from build123d import *

# Parameters (mm, degrees)
F0_W     = 50.8
F0_H     = 25.4
F2_DEPTH = 25.4
F3_DEPTH = 6.35


with BuildPart() as f2:
    # F0 (on Front) → F2 (new body, symmetric)
    with BuildSketch(Plane.XZ):
        Rectangle(F0_W, F0_H)
    extrude(amount=F2_DEPTH, both=True)

    # F1 (on Front) → F3 (cut, symmetric)
    with BuildSketch(Plane.XZ):
        with BuildLine():
            Line((18.556945, 13.312588), (-18.556941, 13.312588))
            ThreePointArc((-18.556941, 13.312588), (2e-06, 0.164781), (18.556945, 13.312588))
        make_face()
    extrude(amount=F3_DEPTH, both=True, mode=Mode.SUBTRACT)


solid = f2.part
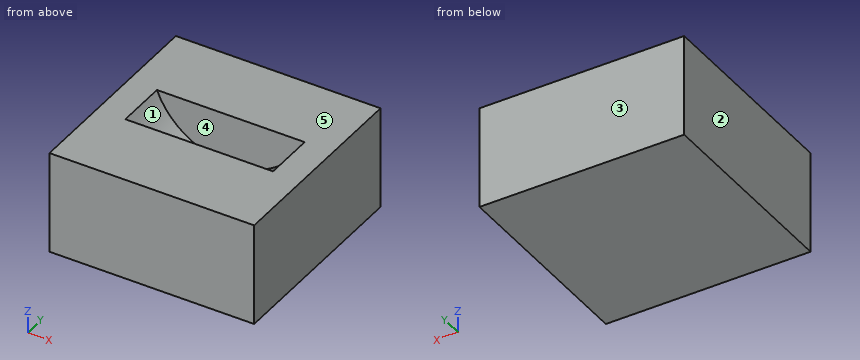
Geometry: final body of the model. Coordinates: model frame, mm. Face numbers are marked on the shaded views. A direction names the side the tool comes from. Round coordinates to 2 decimals unless told otherwise and drop trailing zeros. Order: outer loops, then holes, each group sorted by start corner. A loop starts at its lowest first (then second) coordinate and runs counter-clockwise, first axis right, second up.
Q1. Section C-C, the plane y = 1. Output: boundary loops of the cut face in (x, z).
Result sheet:
outline: (-25.4, -12.7) - (25.4, -12.7) - (25.4, 12.7) - (18.33, 12.7) arc R19.67 cw to (-18.33, 12.7) - (-25.4, 12.7) - close
Q2. Section A-A, the plane z = 11.25. Output: boundary loops of the cut face in (x, y).
Result sheet:
outline: (-25.4, -25.4) - (25.4, -25.4) - (25.4, 25.4) - (-25.4, 25.4) - close; hole (-17.7, -6.35) - (17.7, -6.35) - (17.7, 6.35) - (-17.7, 6.35) - close
Q3. Material intervals for probe 1 along Y at (x, z) = (6, 10.5); probe 2 along X at (y, z) = (6, 6.25); probe 3 along Z at (x, y) = (4, 4), sorted ascending.
Result sheet:
probe 1: y = -25.4 to -6.35, 6.35 to 25.4
probe 2: x = -25.4 to -14.23, 14.23 to 25.4
probe 3: z = -12.7 to 0.58
Q4. Section B-B, the plane x = -5. Output: boundary loops of the cut face in (y, z).
Result sheet:
outline: (-25.4, -12.7) - (25.4, -12.7) - (25.4, 12.7) - (6.35, 12.7) - (6.35, 0.81) - (-6.35, 0.81) - (-6.35, 12.7) - (-25.4, 12.7) - close
Q5. Section D-D, the plane z = 7.5. Output: boundary loops of the cut face in (x, y), and give its area (3 significant figures).
Result sheet:
outline: (-25.4, -25.4) - (25.4, -25.4) - (25.4, 25.4) - (-25.4, 25.4) - close; hole (-15.32, -6.35) - (15.32, -6.35) - (15.32, 6.35) - (-15.32, 6.35) - close
area: 2,190 mm2
Q6. Mould query, pull axis Y, two halves, no side actions, for the marked faces 3, 4 and 5. Classes: released by +Y, released by -Y, zero draft, split by the parting line, or undercut.
Result sheet:
face 3: released by +Y
face 4: undercut
face 5: zero draft
Q7. Access query for the marked faces 1 and 2. Directions: +Z, -Z, +X, -X, +Y, -Y. A direction counts if a zero-diameter tool reaches every point of the face in a straight line with its end or side. Return the directions, or none.
Result sheet:
face 1: +Z
face 2: +Z, -Z, -X, +Y, -Y
